Autodesk Inventor part; units mm, degrees
ref_plane "YZ Plane" through (0, 0, 0) normal (1, 0, 0) x (0, 1, 0)
ref_plane "XZ Plane" through (0, 0, 0) normal (0, 1, 0) x (-1, 0, 0)
ref_plane "XY Plane" through (0, 0, 0) normal (0, 0, 1) x (1, 0, 0)
sketch "Esboço1" plane through (0, 0, 0) normal (0, 0, 1) x (1, 0, 0)
  arc A0 (19, -10) -> (20, -9) centre (19, -9) ccw
  line L0 (20, -4.8) -> (20, -9)
  line L1 (18.2, -3) -> (20, -4.8)
  line L2 (18.2, -5.5) -> (18.2, -3)
  line L3 (16.5607, -5.5) -> (18.2, -5.5)
  line L4 (14, -2.9393) -> (16.5607, -5.5)
  line L5 (14, -0.3) -> (14, -2.9393)
  line L6 (13.7, 0) -> (14, -0.3)
  line L7 (14, 0.3) -> (13.7, 0)
  line L8 (14, 2.9393) -> (14, 0.3)
  line L9 (16.5607, 5.5) -> (14, 2.9393)
  line L10 (18.2, 5.5) -> (16.5607, 5.5)
  line L11 (18.2, 3) -> (18.2, 5.5)
  line L12 (20, 4.8) -> (18.2, 3)
  line L13 (20, 9) -> (20, 4.8)
  arc A1 (20, 9) -> (19, 10) centre (19, 9) ccw
  line L14 (14.8, 10) -> (19, 10)
  line L15 (13, 8.2) -> (14.8, 10)
  line L16 (15.5, 8.2) -> (13, 8.2)
  line L17 (15.5, 6.5607) -> (15.5, 8.2)
  line L18 (12.9393, 4) -> (15.5, 6.5607)
  line L19 (10.3, 4) -> (12.9393, 4)
  line L20 (10, 3.7) -> (10.3, 4)
  line L21 (9.7, 4) -> (10, 3.7)
  line L22 (7.0607, 4) -> (9.7, 4)
  line L23 (4.5, 6.5607) -> (7.0607, 4)
  line L24 (4.5, 8.2) -> (4.5, 6.5607)
  line L25 (7, 8.2) -> (4.5, 8.2)
  line L26 (5.2, 10) -> (7, 8.2)
  line L27 (-5.2, 10) -> (5.2, 10)
  line L28 (-7, 8.2) -> (-5.2, 10)
  line L29 (-4.5, 8.2) -> (-7, 8.2)
  line L30 (-4.5, 6.5607) -> (-4.5, 8.2)
  line L31 (-7.0607, 4) -> (-4.5, 6.5607)
  line L32 (-9.7, 4) -> (-7.0607, 4)
  line L33 (-10, 3.7) -> (-9.7, 4)
  line L34 (-10.3, 4) -> (-10, 3.7)
  line L35 (-12.9393, 4) -> (-10.3, 4)
  line L36 (-15.5, 6.5607) -> (-12.9393, 4)
  line L37 (-15.5, 8.2) -> (-15.5, 6.5607)
  line L38 (-13, 8.2) -> (-15.5, 8.2)
  line L39 (-14.8, 10) -> (-13, 8.2)
  line L40 (-19, 10) -> (-14.8, 10)
  arc A2 (-19, 10) -> (-20, 9) centre (-19, 9) ccw
  line L41 (-20, 4.8) -> (-20, 9)
  line L42 (-18.2, 3) -> (-20, 4.8)
  line L43 (-18.2, 5.5) -> (-18.2, 3)
  line L44 (-16.5607, 5.5) -> (-18.2, 5.5)
  line L45 (-14, 2.9393) -> (-16.5607, 5.5)
  line L46 (-14, 0.3) -> (-14, 2.9393)
  line L47 (-13.7, 0) -> (-14, 0.3)
  line L48 (-14, -0.3) -> (-13.7, 0)
  line L49 (-14, -2.9393) -> (-14, -0.3)
  line L50 (-16.5607, -5.5) -> (-14, -2.9393)
  line L51 (-18.2, -5.5) -> (-16.5607, -5.5)
  line L52 (-18.2, -3) -> (-18.2, -5.5)
  line L53 (-20, -4.8) -> (-18.2, -3)
  line L54 (-20, -9) -> (-20, -4.8)
  arc A3 (-20, -9) -> (-19, -10) centre (-19, -9) ccw
  line L55 (-14.8, -10) -> (-19, -10)
  line L56 (-13, -8.2) -> (-14.8, -10)
  line L57 (-15.5, -8.2) -> (-13, -8.2)
  line L58 (-15.5, -6.5607) -> (-15.5, -8.2)
  line L59 (-12.9393, -4) -> (-15.5, -6.5607)
  line L60 (-10.3, -4) -> (-12.9393, -4)
  line L61 (-10, -3.7) -> (-10.3, -4)
  line L62 (-9.7, -4) -> (-10, -3.7)
  line L63 (-7.0607, -4) -> (-9.7, -4)
  line L64 (-4.5, -6.5607) -> (-7.0607, -4)
  line L65 (-4.5, -8.2) -> (-4.5, -6.5607)
  line L66 (-7, -8.2) -> (-4.5, -8.2)
  line L67 (-5.2, -10) -> (-7, -8.2)
  line L68 (5.2, -10) -> (-5.2, -10)
  line L69 (7, -8.2) -> (5.2, -10)
  line L70 (4.5, -8.2) -> (7, -8.2)
  line L71 (4.5, -6.5607) -> (4.5, -8.2)
  line L72 (7.0607, -4) -> (4.5, -6.5607)
  line L73 (9.7, -4) -> (7.0607, -4)
  line L74 (10, -3.7) -> (9.7, -4)
  line L75 (10.3, -4) -> (10, -3.7)
  line L76 (12.9393, -4) -> (10.3, -4)
  line L77 (15.5, -6.5607) -> (12.9393, -4)
  line L78 (15.5, -8.2) -> (15.5, -6.5607)
  line L79 (13, -8.2) -> (15.5, -8.2)
  line L80 (14.8, -10) -> (13, -8.2)
  line L81 (19, -10) -> (14.8, -10)
  line L82 (-2.7, 8.2) -> (2.7, 8.2)
  line L83 (2.7, 8.2) -> (2.7, 6.2393)
  line L84 (2.7, 6.2393) -> (6, 2.9393)
  line L85 (6, 2.9393) -> (6, -2.9393)
  line L86 (6, -2.9393) -> (2.7, -6.2393)
  line L87 (2.7, -6.2393) -> (2.7, -8.2)
  line L88 (2.7, -8.2) -> (-2.7, -8.2)
  line L89 (-2.7, -8.2) -> (-2.7, -6.2393)
  line L90 (-2.7, -6.2393) -> (-6, -2.9393)
  line L91 (-6, -2.9393) -> (-6, 2.9393)
  line L92 (-6, 2.9393) -> (-2.7, 6.2393)
  line L93 (-2.7, 6.2393) -> (-2.7, 8.2)
  circle A4 centre (10, 0) radius 2.5
  circle A5 centre (-10, 0) radius 2.5
  point P0 (0, 0)
  point P1 (0, 0)
extrude "Extrusão1" add sketch "Esboço1" along normal blind 10
properties part number "PERFIL_ESTRUTURAL_20X40"
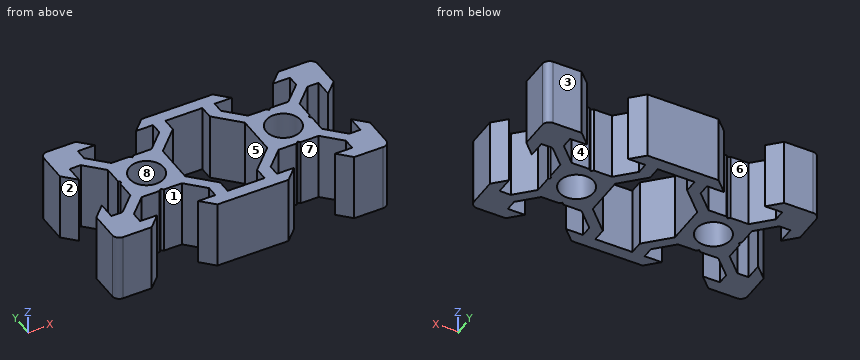
Verification items for the finished model (mm, model axes). Face numbers are marked on the shaded views. A direction names the side the tool comes from. Round coordinates to 2 decimals unless told otherwise and drop trailing zeros. Loops run counter-clockwise (first coordinate to the right, second up) from the corner with the lowest first, then second, coordinate; pieces in that order, holes last. Notation, with made-up numbers: (13.5, 34.5) - (72.5, 34.5) arc R16 ccw to (72.5, 53.5) - close; hole circle Ø3 at (32.5, -2). An arc over 180 degrees is marked (long way). Use a Markdown table: item, result. Add a question column.
1. Section check A-A, the plane x = 16. Record the boundary of the cut face in (y, z).
2. Thickness scan on probe 1 along X at (y, z) = (7, 7.25); probe 2 along Y at (x, z) = (-17.5, 0.5); probe 3 along X at (y, z) = (9.25, 1.25). Record the ranges inside material, lowest first. Write a range as [from, to].
3. Section check B-B, the plane z = 0.5. Give the number of separate pieces and of enclosed holes in the cut face, plus the area to 3 significant figures.
4. Access from +Z, -Z, +X, -X, +Y, -Y to the whole of each face (thin tool, end or side, straight path). Record for the marked faces 1, 2, 3, 4 and 5.
5. Gauge pin test, flat ends, axial feed: pin 1 (2 mm diameter, centred on y = -4.5, z = 5.5, fed in from +X); pin 2 (1.3 mm diameter, centred on x = -8.5, z = 2.5, fed in from -Y); pin 3 (1.2 mm diameter, centred on x = -6.5, z = 3, fed in from +Y); pin 4 (1 mm diameter, centred on y = -3, z = 5, fed in from +X). Record the tip position at first contact, or that the pin passes through.
6. Release check for a two-part mould opening along Y. For the marked faces 6, 7 and 8 record: released by +Y, released by -Y, zero draft, split by the parting line, or undercut.
Checks:
| question | item | result |
|---|---|---|
| 1 | outline | (-10, 0) - (-4.94, 0) - (-4.94, 10) - (-10, 10) - close; (4.94, 0) - (10, 0) - (10, 10) - (4.94, 10) - close |
| 2 | probe 1 | x = [-20, -15.5], [-4.5, -2.7], [2.7, 4.5], [15.5, 20] |
| 2 | probe 2 | y = [-10, -5.5], [5.5, 10] |
| 2 | probe 3 | x = [-19.97, -14.05], [-5.95, 5.95], [14.05, 19.97] |
| 3 | separate pieces | 1 |
| 3 | enclosed holes | 3 |
| 3 | area | 288 mm^2 |
| 4 | face 1 | +Z, -Z, -Y |
| 4 | face 2 | +Z, -Z, -X |
| 4 | face 3 | +Z, -Z, +X, -X, +Y |
| 4 | face 4 | +Z, -Z, +Y |
| 4 | face 5 | +Z, -Z |
| 5 | pin 1 | stops at x = 20 |
| 5 | pin 2 | stops at y = -4 |
| 5 | pin 3 | stops at y = 9.3 |
| 5 | pin 4 | stops at x = 18.7 |
| 6 | face 6 | released by +Y |
| 6 | face 7 | released by -Y |
| 6 | face 8 | undercut |
